CAD build for the part. Positions are in the model's coordinates, mm. Face numbers are marked on the shaded views. A direction names the side the tool comes from. Round coordinates to 2 decimals unless told otherwise and drop trailing zeros. Order: outer loops, then holes, each group sorted by start corner. A loop starts at its lowest first (then second) coordinate and runs counter-clockwise, first axis right, second up. Notation, with made-up numbers: (13, -34) -> (32, -34) arc R28 ccw to (32, -5) -> close; hole circle Ø2 at (80, -3.75). An arc over 180 degrees is marked (long way). Return JSON: item names as keys, results as strings. Group by question number.
Q1. Cut at C-C (x = 3.5). Write the cut outline in (y, z), then the cut area to 3 significant figures.
Q2. Cut at B-B (x = -22). Write the cut outline in (y, z).
Q3. Mould opens along X. For the marked faces 3, 4 and 5 say: +X half, -X half, draft (parallel to the pull), parting line (faces both ways), or undercut.
Q4. Which spindle directions (+Z, -Z, +X, -X, +Y, -Y) get a long thin tool onto all of the face, cutting with end or side? Do the marked faces 1 and 2. Say none if no direction does.
Q5. Flat gauge pins, fed straight in: pin 1 (4 mm diameter, centred on x = 67, z = 12, fed in from +Y); pin 2 (1.6 mm diameter, centred on x = 8, y = 3, fed in from -Z); pin 3 (1.5 mm diameter, centred on x = -33.5, z = 10.5, fed in from +Y); pin 4 (11 mm diameter, centred on x = 63, z = 15, fed in from -Y). Where does each tip first touch, or does it go through?
Q6. Cut at A-A (y = -4.5). Write the cut outline in (x, z).
Q7. Probe line 1 along Z through (x, y) = (-42, 8.75); line 2 along Y through (x, z) = (-10, 12.75); line 3 along Y through (x, z) = (97, 8.25). List the from-to ranges inside material, lowest first.
Autodesk Inventor part; units mm, degrees
ref_plane "YZ Plane" through (0, 0, 0) normal (1, 0, 0) x (0, 1, 0)
ref_plane "XZ Plane" through (0, 0, 0) normal (0, 1, 0) x (-1, 0, 0)
ref_plane "XY Plane" through (0, 0, 0) normal (0, 0, 1) x (1, 0, 0)
sketch "スケッチ2" plane through (0, 0, 0) normal (0, 0, 1) x (1, 0, 0)
  arc A0 (-18.0723, 8.4646) -> (-44.4977, 8.2149) centre (-30.9427, -27.8877) ccw
  arc A1 (-18.0723, 8.4646) -> (17.6933, 1.1527) centre (26.0163, 132.9927) ccw
  arc A2 (99.6933, 1.1527) -> (115.4364, 3.2181) centre (99.6933, 62.1838) ccw
  arc A3 (-44.4977, 8.2149) -> (-72.801, -6.8342) centre (-0.878, -107.9623) ccw
  line L0 (17.6933, 1.1527) -> (99.6933, 1.1527)
  arc A4 (-43.7244, 6.1553) -> (-71.526, -8.627) centre (-0.878, -107.9623) ccw
  arc A5 (-18.8066, 6.3908) -> (-43.7244, 6.1553) centre (-30.9427, -27.8877) ccw
  arc A6 (-18.8066, 6.3908) -> (17.6242, -1.0473) centre (26.0163, 132.9927) ccw
  line L1 (17.6242, -1.0473) -> (99.6933, -1.0473)
  arc A7 (99.6933, -1.0473) -> (116.0039, 1.0926) centre (99.6933, 62.1838) ccw
  line L2 (-72.801, -6.8342) -> (-71.526, -8.627)
  line L3 (115.4364, 3.2181) -> (116.0039, 1.0926)
  point P0 (0, 0)
  dimension "d19" = 82
  dimension "d26" = 132.1025
  dimension "d27" = 38.5634
  dimension "d28" = 124.096
  dimension "d29" = 14.842
  dimension "d30" = 40.075
  dimension "d31" = 15.884
  dimension "d32" = 14.949
  dimension "d33" = 61.0311
  dimension "d34" = 2.2
extrude "押し出し2" add sketch "スケッチ2" along normal blind 24.32
sketch "スケッチ3" plane through (17.6242, -1.0473, 0) normal (0, -1, 0) x (1, 0, 0)
  line L0 (98.3797, 0) -> (98.3797, 24.32)
  arc A0 (-45.5784, 24.32) -> (-58.4546, 24.1908) centre (-45.5784, -617.2518) ccw
  line L1 (-61.3487, 24.32) -> (-36.4308, 24.32)
  arc A1 (-27.6481, 17.7751) -> (-45.5784, 24.32) centre (-45.5784, -3.5132) ccw
  arc A2 (-27.6481, 17.7751) -> (-21.3876, 15.4513) centre (-21.2803, 25.3354) ccw
  arc A3 (95.2752, 19.5094) -> (3.1956, 15.4513) centre (209.2083, -3612.3091) ccw
  line L2 (97.8122, 0) -> (97.8122, 24.32)
  arc A4 (98.3797, 12.16) -> (95.2752, 19.5094) centre (88.128, 12.16) ccw
  line L3 (-21.3876, 15.4513) -> (3.1956, 15.4513)
  line L4 (-90.4253, 0) -> (-90.4253, 24.32)
  line L5 (-58.4546, 24.1908) -> (-90.4253, 20.6993)
  line L6 (-90.4253, 20.6993) -> (-58.4546, 18.5366)
  line L7 (-58.4546, 18.5366) -> (-90.4253, 14.6253)
  line L8 (-90.4253, 14.6253) -> (-58.4546, 12.16)
  line L9 (-58.4546, 12.16) -> (98.3797, 12.16)
  arc A5 (-58.4546, 0.1292) -> (-45.5784, 0) centre (-45.5784, 641.5718) ccw
  arc A6 (-45.5784, 0) -> (-27.6481, 6.5449) centre (-45.5784, 27.8332) ccw
  arc A7 (-21.3876, 8.8687) -> (-27.6481, 6.5449) centre (-21.2803, -1.0154) ccw
  arc A8 (3.1956, 8.8687) -> (95.2752, 4.8106) centre (209.2083, 3636.6291) ccw
  arc A9 (95.2752, 4.8106) -> (98.3797, 12.16) centre (88.128, 12.16) ccw
  line L10 (-21.3876, 8.8687) -> (3.1956, 8.8687)
  line L11 (-58.4546, 0.1292) -> (-90.4253, 3.6207)
  line L12 (-90.4253, 3.6207) -> (-58.4546, 5.7834)
  line L13 (-58.4546, 5.7834) -> (-90.4253, 9.6947)
  line L14 (-90.4253, 9.6947) -> (-58.4546, 12.16)
  point P0 (97.8122, 12.16)
  point P1 (97.8122, 8.7964)
  point P2 (97.8122, 15.5236)
extrude "押し出し3" cut sketch "スケッチ3" along normal mid plane 24.32 contours A1 A2 L3 A3 A4 L2 L9 L8 L7 L6 L5 A0 | L14 L9 L2 A9 A8 L10 A7 A6 A5 L11 L12 L13 keep common part
sketch "スケッチ4" plane through (17.6242, -1.0473, 8.8687) normal (0, -1, 0) x (1, 0, 0)
  line L0 (97.8122, 6.6548) -> (97.8122, -0.0723)
  point P0 (-17.6242, -8.8687)
  point P1 (74.8122, 3.2913)
  point P2 (97.8122, 3.2913)
  point P3 (24.8122, 3.2913)
  dimension "d39" = 23
  dimension "d47" = 50
hole "穴1" at (92.4364, -1.0473, 12.16) at (42.4364, -1.0473, 12.16) direction (0, 1, 0) diameter 3.4 end through all
properties part number "fork" material "ポリスチレン"
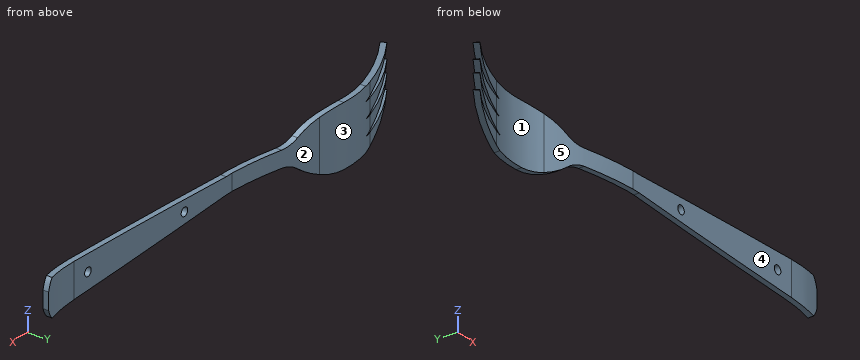
Solution:
{
 "1": {"outline": "(0.59, 8.87) -> (2.82, 8.87) -> (2.82, 15.45) -> (0.59, 15.45) -> close", "area": "14.7 mm²"},
 "2": {"outline": "(7.36, 0.64) -> (9.62, 0.64) -> (9.62, 23.68) -> (7.36, 23.68) -> close"},
 "3": {"face 3": "parting line", "face 4": "draft", "face 5": "undercut"},
 "4": {"face 1": "+Z, -Z, -Y", "face 2": "+Z, -Z, +Y"},
 "5": {"pin 1": "stops at y = 1.15", "pin 2": "passes through", "pin 3": "stops at y = 10.63", "pin 4": "stops at y = -1.05"},
 "6": {"outline": "(-69.4, 3.25) -> (-65.33, 2.8) -> (-65.33, 4.13) -> (-69.4, 3.85) -> close; (-69.4, 9.28) -> (-65.33, 8.78) -> (-65.33, 10.27) -> (-69.4, 9.96) -> close; (-69.4, 14.36) -> (-65.33, 14.05) -> (-65.33, 15.54) -> (-69.4, 15.04) -> close; (-69.4, 20.47) -> (-65.33, 20.19) -> (-65.33, 21.52) -> (-69.4, 21.07) -> close"},
 "7": {"line 1": "z = 0.26 to 5.7, 5.93 to 12.07, 12.25 to 18.39, 18.62 to 24.06", "line 2": "y = 3.61 to 5.89", "line 3": "y = -1.05 to 1.15"}
}
